Geometry: final body of the model. Coordinates: model frame, mm. Face numbers are marked on the shaded views. A direction names the side the tool comes from. Round coordinates to 2 decimals unless told otherwise and drop trailing zeros. Loops run counter-clockwise (first coordinate to the right, second up) from the corner with the lowest first, then second, coordinate; pieces in that order, holes last. Notation, with made-up numbers: (-27, 32.5) - (17, 32.5) arc R35 ccw to (17, 68.5) - close; hole circle Ø5 at (-10, 77.5). An arc over 180 degrees is marked (long way). Use CSV: the item, a comma, the result in double quotes.
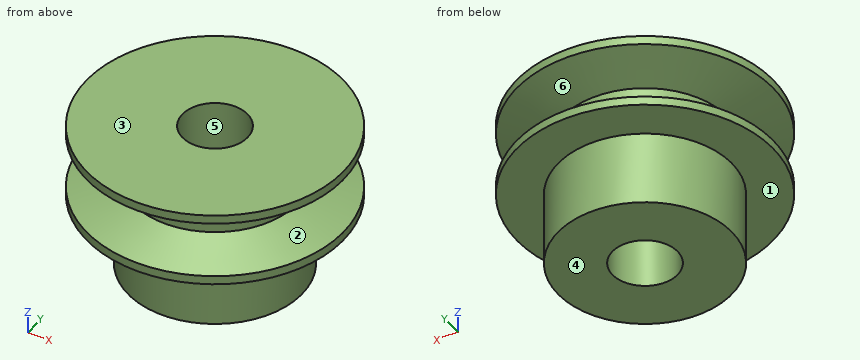
Autodesk Inventor part; units mm, degrees
ref_plane "YZ Plane" through (0, 0, 0) normal (1, 0, 0) x (0, 1, 0)
ref_plane "XZ Plane" through (0, 0, 0) normal (0, 1, 0) x (-1, 0, 0)
ref_plane "XY Plane" through (0, 0, 0) normal (0, 0, 1) x (1, 0, 0)
sketch "Sketch1" plane through (0, 0, 0) normal (0, 0, 1) x (1, 0, 0)
  circle A0 centre (17.8, 18.8069) radius 20
  circle A1 centre (17.8, 18.8069) radius 7.5
  point P0 (0, 0)
  dimension "d0" = 40
  dimension "d1" = 15
extrude "Extrusion1" add sketch "Sketch1" along normal blind 17
sketch "Sketch2" plane through (17.8, 18.8069, 0) normal (0, 0, -1) x (-1, 0, 0)
  point P0 (17.8, -18.8069)
sketch "Sketch3" plane through (17.8, 18.8069, 17) normal (0, 0, 1) x (1, 0, 0)
  circle A0 centre (0, 0) radius 29.5
  point P0 (-17.8, -18.8069)
  dimension "d4" = 59
extrude "Extrusion2" add sketch "Sketch3" along normal blind 5
sketch "Sketch4" plane through (17.8, 18.8069, 17) normal (0, 0, -1) x (-1, 0, 0)
  circle A0 centre (0, 0) radius 8.6163
  point P0 (17.8, -18.8069)
sketch "Sketch5" plane through (17.8, 18.8069, 22) normal (0, 0, 1) x (1, 0, 0)
  circle A0 centre (0, 0) radius 7.5
  point P0 (-17.8, -18.8069)
extrude "Extrusion3" cut sketch "Sketch5" against normal blind 57.5
sketch "Sketch6" plane through (17.8, 18.8069, 17) normal (0, 0, -1) x (-1, 0, 0)
  point P0 (17.8, -18.8069)
sketch "Sketch7" plane through (17.8, 18.8069, 22) normal (0, 0, 1) x (1, 0, 0)
  point P0 (-17.8, -18.8069)
sketch "Sketch8" plane through (17.8, 18.8069, 22) normal (0, 0, 1) x (1, 0, 0)
  circle A0 centre (0, 0) radius 19
  point P0 (-17.8, -18.8069)
  dimension "d9" = 38
extrude "Extrusion4" add sketch "Sketch8" along normal blind 7
sketch "Sketch9" plane through (17.8, 18.8069, 29) normal (0, 0, 1) x (1, 0, 0)
  circle A0 centre (0, 0) radius 29.5
  point P0 (-17.8, -18.8069)
extrude "Extrusion5" add sketch "Sketch9" along normal blind 5
sketch "Sketch10" plane through (17.8, 18.8069, 22) normal (0, 0, -1) x (-1, 0, 0)
  circle A0 centre (0, 0) radius 7.5
  circle A1 centre (0, 0) radius 7.5
  point P0 (17.8, -18.8069)
sketch "Sketch11" plane through (17.8, 18.8069, 34) normal (0, 0, 1) x (1, 0, 0)
  circle A0 centre (0, 0) radius 7.5
  point P0 (-17.8, -18.8069)
extrude "Extrusion6" cut sketch "Sketch11" against normal blind 76.5
chamfer "Chamfer1" distance 3 distance2 10.5 1 edges at (-11.7, 18.8069, 29) measured on face at (47.2043, 16.4331, 32.3333)
chamfer "Chamfer2" distance 3 distance2 10.5 1 edges at (-11.7, 18.8069, 22) measured on face at (47.2043, 16.4331, 20.3333)
properties part number "Polia"
Item 1: Pin query (flat end, axial travel): P1, Ø5, axis at y = -4, z = 6.5, coming from the +X side; P2, Ø12, axis at x = 28.5, z = 17, coming from the +Y side; P3, Ø1, axis at x = 30.5, z = 10, coming from the -Y side; P4, Ø6, axis at y = 29, z = 13, coming from the +X side. Return the tip coordinate at first contact, or that it passes through.
Final values:
P1,"passes through"
P2,"stops at y = 47.93"
P3,"stops at y = 2.96"
P4,"stops at x = 36.46"
Item 2: Section B-B on z = 15. Return the cut outline in (x, y), plus the area to 3 significant figures.
Final values:
outline,"circle Ø40 at (17.8, 18.81); hole circle Ø15 at (17.8, 18.81)"
area,"1,080 mm²"
Item 3: Reachability of the marked faces 1, 2 and 3 from +Z, -Z, +X, -X, +Y, -Y: full face, straight path, thin tool, end or side. Return the list, or none.
Final values:
face 1,"-Z"
face 2,"none"
face 3,"+Z, +X, -X, +Y, -Y"
Item 4: Mould query, pull axis Z, two halves, no side actions, for the marked faces 4, 5 and 6. Classes: released by +Z, released by -Z, zero draft, split by the parting line, or undercut.
Final values:
face 4,"released by -Z"
face 5,"zero draft"
face 6,"undercut"
Item 5: Section C-C on z = 28. Return the cut outline in (x, y), plus the area to 3 significant figures.
Final values:
outline,"circle Ø38 at (17.8, 18.81); hole circle Ø15 at (17.8, 18.81)"
area,"957 mm²"
Item 6: Material intervals for line 1 (Y direction, x = 17.8, z = 12); line 2 (Y direction, x = 17.8, z = 24); line 3 (Z direction, x = 1.5, y = -2), sorted ascending.
Final values:
line 1,"y = -1.19 to 11.31, 26.31 to 38.81"
line 2,"y = -0.19 to 11.31, 26.31 to 37.81"
line 3,"z = 17 to 19.88, 31.12 to 34"
